```python
from build123d import *

# Parameters (mm, degrees)
FILLET3_R           = 25
FILLET4_R           = 25
BOSS_EXTRUDE1_REACH = 317
SKETCH2_R           = 58
SKETCH3_R           = 110
BOSS_EXTRUDE2_DEPTH = 20
CUT_EXTRUDE1_REACH  = 337
SKETCH4_R           = 38
SKETCH5_R           = 9
CUT_EXTRUDE2_DEPTH  = 20
CIRPATTERN1_COUNT   = 6
SKETCH6_R           = 9
CUT_EXTRUDE3_DEPTH  = 20
CIRPATTERN2_COUNT   = 6
SKETCH7_R           = 9
CUT_EXTRUDE4_DEPTH  = 20
CIRPATTERN3_COUNT   = 6
FILLET6_R           = 10


with BuildPart() as part:
    # Sketch1 → Revolve1 (revolve)
    with BuildSketch(Plane.XY, mode=Mode.PRIVATE) as revolve1_sk:
        with BuildLine():
            Line((38, 0), (110, 0))
            Line((110, 0), (110, 20))
            Line((110, 20), (58, 20))
            Line((58, 20), (58, 74))
            Line((58, 74), (90, 74))
            Line((90, 74), (90, 254))
            Line((90, 254), (135, 254))
            Line((135, 254), (135, 274))
            Line((135, 274), (79, 274))
            Line((79, 274), (79, 268))
            Line((79, 268), (70, 268))
            Line((70, 268), (70, 106))
            ThreePointArc((70, 106), (67.656854249, 100.343145751), (62, 98))
            Line((62, 98), (60, 98))
            Line((60, 98), (60, 88))
            Line((60, 88), (46, 88))
            Line((46, 88), (46, 34))
            Line((46, 34), (38, 34))
            Line((38, 34), (38, 0))
        make_face()
    revolve(revolve1_sk.sketch.rotate(Axis((0, 0, 0), (0, 1, 0)), 90), axis=Axis((0, 0, 0), (0, 1, 0)))  # turned: the seam where the file's is

    # Fillet3
    fillet3_edges = [part.edges().sort_by_distance(p)[0] for p in [
        (0, 74, 90),
    ]]
    fillet(fillet3_edges, radius=FILLET3_R)

    # Fillet4
    fillet4_edges = [part.edges().sort_by_distance(p)[0] for p in [
        (0, 74, 58),
    ]]
    fillet(fillet4_edges, radius=FILLET4_R)

    # Sketch2 → Boss-Extrude1 (add, up to next)
    with BuildSketch(Plane(origin=(180, 0, 0), x_dir=(0, 0, -1), z_dir=(1, 0, 0)), mode=Mode.PRIVATE) as boss_extrude1_sk1:
        with Locations((0, 132)):
            Circle(SKETCH2_R)
    boss_extrude1_tool1 = extrude(boss_extrude1_sk1.sketch, amount=-BOSS_EXTRUDE1_REACH, mode=Mode.PRIVATE) - part.part
    add(boss_extrude1_tool1.solids().sort_by_distance((180, 132, 0))[0])

    # Sketch3 → Boss-Extrude2 (add)
    with BuildSketch(Plane(origin=(180, 0, 0), x_dir=(0, 0, -1), z_dir=(1, 0, 0))):
        with Locations((0, 132)):
            Circle(SKETCH3_R)
    extrude(amount=BOSS_EXTRUDE2_DEPTH)

    # Sketch4 → Cut-Extrude1 (cut, up to next)
    with BuildSketch(Plane(origin=(200, 0, 0), x_dir=(0, 0, -1), z_dir=(1, 0, 0)), mode=Mode.PRIVATE) as cut_extrude1_sk1:
        with Locations((0, 132)):
            Circle(SKETCH4_R)
    cut_extrude1_tool1 = extrude(cut_extrude1_sk1.sketch, amount=-CUT_EXTRUDE1_REACH, mode=Mode.PRIVATE) & part.part
    add(cut_extrude1_tool1.solids().sort_by_distance((200, 132, 0))[0], mode=Mode.SUBTRACT)

    # Sketch5 → Cut-Extrude2 (cut)
    with BuildSketch(Plane(origin=(0, 274, 0), x_dir=(1, 0, 0), z_dir=(0, 1, 0))):
        with Locations(Location((0, 112, 0), (0, 0, 270))):  # turned: the seam where the file's is
            Circle(SKETCH5_R)
    cut_extrude2 = extrude(amount=-CUT_EXTRUDE2_DEPTH, mode=Mode.SUBTRACT)

    # CirPattern1: Cut-Extrude2 ×6 about axis
    cirpattern1_axis = Axis((0, 0, 0), (0, 1, 0))
    for i in range(1, CIRPATTERN1_COUNT):
        add(cut_extrude2.rotate(cirpattern1_axis, i * 360 / CIRPATTERN1_COUNT), mode=Mode.SUBTRACT)

    # Sketch6 → Cut-Extrude3 (cut)
    with BuildSketch(Plane(origin=(200, 0, 0), x_dir=(0, 0, -1), z_dir=(1, 0, 0))):
        with Locations((0, 218)):
            Circle(SKETCH6_R)
    cut_extrude3 = extrude(amount=-CUT_EXTRUDE3_DEPTH, mode=Mode.SUBTRACT)

    # CirPattern2: Cut-Extrude3 ×6 about axis
    cirpattern2_axis = Axis((0, 132, 0), (1, 0, 0))
    for i in range(1, CIRPATTERN2_COUNT):
        add(cut_extrude3.rotate(cirpattern2_axis, i * 360 / CIRPATTERN2_COUNT), mode=Mode.SUBTRACT)

    # Sketch7 → Cut-Extrude4 (cut)
    with BuildSketch(Plane(origin=(0, 20, 0), x_dir=(1, 0, 0), z_dir=(0, 1, 0))):
        with Locations(Location((0, 88, 0), (0, 0, 270))):  # turned: the seam where the file's is
            Circle(SKETCH7_R)
    cut_extrude4 = extrude(amount=-CUT_EXTRUDE4_DEPTH, mode=Mode.SUBTRACT)

    # CirPattern3: Cut-Extrude4 ×6 about axis
    cirpattern3_axis = Axis((0, 0, 0), (0, 1, 0))
    for i in range(1, CIRPATTERN3_COUNT):
        add(cut_extrude4.rotate(cirpattern3_axis, i * 360 / CIRPATTERN3_COUNT), mode=Mode.SUBTRACT)

    # Fillet6
    fillet6_edges = [part.edges().sort_by_distance(p)[0] for p in [
        (0, 20, 58),
    ]]
    fillet(fillet6_edges, radius=FILLET6_R)


solid = part.part
```
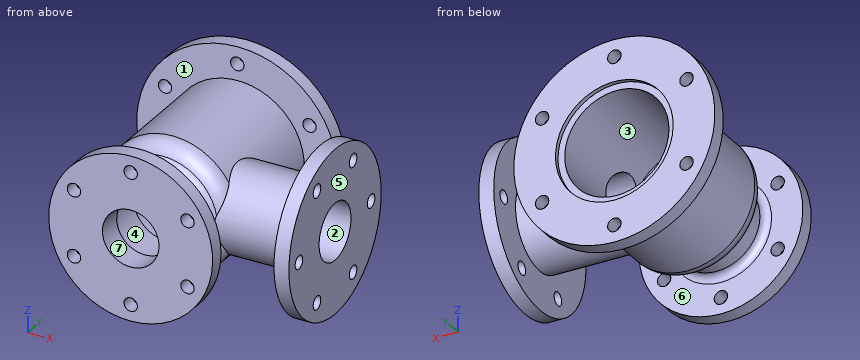
The listing builds one solid part. Answer for the finished solid, in the listing's coordinates (mm). Face numbers are marked on the shaded views. A direction names the side the tool comes from. Coordinates: 2 decimals unless noted, no trailing zeros. Write each loop counter-clockwise with the first axis right and the second up, starting at its lowest first coordinate (ties: lowest second). Pieces come first, ordered by that corner, then holes.
Q1. Section D-D, the plane y = 237.5 is taken. Write down the section's boundary in (x, z), then the cut area to 3 significant figures.
Returned:
outline: circle Ø180 at (0, 0); (180, -31.14) - (200, -31.14) - (200, 31.14) - (180, 31.14) - close; hole circle Ø140 at (0, 0)
area: 11,300 mm2
Q2. Given P1, Ø16, axis at y = 175, z = 74.48, coming from the +X side; P2, Ø5, axis at x = -0.5, y = 188.5, coming from the +Z side; P3, Ø11, axis at x = -96.99, z = -56, coming from the +Y side, each flat-ended and moving along its own axis, determine where each tip first touches the part or whether it passes through.
Returned:
P1: stops at x = 60.67
P2: stops at z = 90
P3: stops at y = 20
Q3. Section A-A, the plane x = 95 is taken. Write down the section's boundary in (y, z).
Returned:
outline: (0, -55.45) - (20, -55.45) - (20, 55.45) - (0, 55.45) - close; circle Ø116 at (132, 0); (254, -95.92) - (274, -95.92) - (274, -64.78) - (254, -64.78) - close; (254, -47.22) - (274, -47.22) - (274, 47.22) - (254, 47.22) - close; (254, 64.78) - (274, 64.78) - (274, 95.92) - (254, 95.92) - close; hole circle Ø76 at (132, 0)
Q4. The mould has two halves that part along X. Classify the marked faces 4, 5, 6 and 7: released by +X, released by -X, zero draft, split by the parting line, or undercut.
Returned:
face 4: undercut
face 5: released by +X
face 6: zero draft
face 7: undercut
Q5. Section B-B, the plane y = 46 is taken. Write down the section's boundary in (x, z).
Returned:
outline: circle Ø116 at (0, 0); (180, -68.59) - (200, -68.59) - (200, -9) - (180, -9) - close; (180, 9) - (200, 9) - (200, 68.59) - (180, 68.59) - close; hole circle Ø92 at (0, 0)
Q6. Section C-C, the plane x = -97 is taken. Write down the section's boundary in (y, z), then the cut area to 3 significant figures.
Returned:
outline: (0, -51.87) - (20, -51.87) - (20, 51.87) - (0, 51.87) - close; (254, -93.89) - (274, -93.89) - (274, -65) - (254, -65) - close; (254, -47) - (274, -47) - (274, 47) - (254, 47) - close; (254, 65) - (274, 65) - (274, 93.89) - (254, 93.89) - close
area: 5,110 mm2
Q7. Find the intervals of material crossed by line 1 along Y through (x, z) = (194.25, 0); line 2 along Y through (x, z) = (86.5, 61.5); line 3 along X through (y, z) = (62, -8), in increasing order.
Returned:
line 1: y = 22 to 37, 55 to 94, 170 to 209, 227 to 242
line 2: y = 0 to 20, 254 to 274
line 3: x = -59.4 to -45.3, 45.3 to 59.4, 180 to 200
Q8. Which of the six approach directions +Z, -Z, +X, -X, +Y, -Y give full straight-line access (tool end or side, diameter ignored) to the marked faces 1, 2 and 3?
Returned:
face 1: none
face 2: +X
face 3: +Y
